Work out the finished part from the listing and answer in its coordinate system (mm). A direction names the side the tool comes from. Coordinates: 2 decimals unless noted, no trailing zeros. Order: outer loops, then holes, each group sorted by start corner. A loop starts at its lowest first (then second) coordinate and runs counter-clockwise, first axis right, second up. Notation, with made-up numbers: (48, -2) -> (90, -2) arc R22 cw to (90, 32) -> close; hole circle Ø2 at (-10.75, -21). An arc over 180 degrees is marked (long way). Answer as CSV lines item,"result". Start each with the question number.
Item 1: Section C-C (z = 33) is taken. Write down the section's boundary in (x, y).
Item 2: Section A-A (y = 1049) is taken. Write down the section's boundary in (x, z), then the cut area to 3 significant figures.
Item 3: Straight lines are drawn through the part: L1, parallel to Y at x = 632.5, z = 37.5; L2, parallel to Y at x = 601, z = 47; L3, parallel to Z at x = 624, y = 1052. For each, find the intervals that lie inside material, in ascending order.
Item 4: Which of the six approach directions +Z, -Z, +X, -X, +Y, -Y give full straight-line access (tool end or side, diameter ignored) to faces 4 (the face through (618, 1025, 53.172)), 5 (the face through (911, 899.027, 77))?
Item 5: For a pull along Y with two mould halves and no side action, classify faces 1 (the face through (911, 1026, 3.172)), 2 (the face through (911, 1149.027, 77)), 3 (the face through (672.11, 1074.72, 27.82)) as pulls with the +Y half, pulls with the -Y half, needs draft (parallel to the pull), parting line crosses it, or undercut.
Item 6: Section B-B (x = 560) is taken. Write down the section's boundary in (y, z).
```python
from build123d import *

# Parameters (mm, degrees)
CROQUIS2_W              = 850
CROQUIS2_H              = 250
SALIENTE_EXTRUIR1_DEPTH = 150
CROQUIS3_R              = 75
CORTAR_EXTRUIR1_DEPTH   = 50


with BuildPart() as part:
    # Croquis2 → Saliente-Extruir1 (new body)
    with BuildSketch(Plane.XY.offset(3.171613416)):
        with Locations((916.834843653, 1024.026997685)):
            Rectangle(CROQUIS2_W, CROQUIS2_H)
    extrude(amount=SALIENTE_EXTRUIR1_DEPTH)

    # Croquis3 → Cortar-Extruir1 (cut)
    with BuildSketch(Plane(origin=(0, 0, 3.171613416), x_dir=(-1, 0, 0), z_dir=(0, 0, -1))):
        with Locations((-616.834843653, 1024.026997685)):
            Circle(CROQUIS3_R)
    extrude(amount=-CORTAR_EXTRUIR1_DEPTH, mode=Mode.SUBTRACT)


solid = part.part
```
Checked values:
1,outline,"(491.83, 899.03) -> (1341.83, 899.03) -> (1341.83, 1149.03) -> (491.83, 1149.03) -> close; hole circle Ø150 at (616.83, 1024.03)"
2,outline,"(491.83, 3.17) -> (546.11, 3.17) -> (546.11, 53.17) -> (687.56, 53.17) -> (687.56, 3.17) -> (1341.83, 3.17) -> (1341.83, 153.17) -> (491.83, 153.17) -> close"
2,area,"120,000 mm^2"
3,L1,"y = 899.03 to 950.68, 1097.37 to 1149.03"
3,L2,"y = 899.03 to 950.72, 1097.34 to 1149.03"
3,L3,"z = 53.17 to 153.17"
4,face 4,"-Z"
4,face 5,"+Z, -Z, +X, -X, -Y"
5,face 1,"needs draft"
5,face 2,"pulls with the +Y half"
5,face 3,"undercut"
6,outline,"(899.03, 3.17) -> (975.09, 3.17) -> (975.09, 53.17) -> (1072.96, 53.17) -> (1072.96, 3.17) -> (1149.03, 3.17) -> (1149.03, 153.17) -> (899.03, 153.17) -> close"
